Autodesk Inventor part; units mm, degrees
ref_plane "YZ Plane" through (0, 0, 0) normal (1, 0, 0) x (0, 1, 0)
ref_plane "XZ Plane" through (0, 0, 0) normal (0, 1, 0) x (-1, 0, 0)
ref_plane "XY Plane" through (0, 0, 0) normal (0, 0, 1) x (1, 0, 0)
sketch "Sketch1" plane through (0, 0, 0) normal (0, 1, 0) x (-1, 0, 0)
  line L0 (0, 0) -> (9.525, 0)
  line L1 (9.525, 0) -> (9.525, -28.575)
  line L2 (9.525, -28.575) -> (0, -28.575)
  line L3 (0, -28.575) -> (0, 0)
  circle A0 centre (3.175, -4.0894) radius 1.27
  circle A1 centre (3.175, -24.4856) radius 1.27
  dimension "d0" = 9.525
  dimension "d1" = 28.575
  dimension "d2" = 2.54
  dimension "d3" = 2.54
  dimension "d4" = 20.3962
  dimension "d5" = 4.0894
  dimension "d6" = 6.35
extrude "Extrusion1" add sketch "Sketch1" along normal blind 3.175
sketch "Sketch2" plane through (-9.525, 0, -28.575) normal (-1, 0, 0) x (0, 0, 1)
  line L0 (28.575, 0) -> (0, 0)
  line L1 (28.575, 0) -> (28.575, 3.175)
  line L2 (0, 3.175) -> (28.575, 3.175)
  line L3 (0, 0) -> (0, 3.175)
  line L4 (28.575, 3.175) -> (0, 3.175)
  line L5 (28.575, 3.175) -> (0, 3.175)
  line L6 (0, 3.175) -> (0, -6.35)
  line L7 (0, -6.35) -> (28.575, -6.35)
  line L8 (28.575, -6.35) -> (28.575, 3.175)
  point P0 (28.575, 0)
  dimension "d9" = 9.525
extrude "Extrusion2" add sketch "Sketch2" along normal blind 1.5875
sketch "Sketch3" plane through (-9.525, 0, -28.575) normal (1, 0, 0) x (0, 0, -1)
  line L0 (-28.575, 0) -> (0, 0)
  line L1 (-28.575, -6.35) -> (-28.575, 0)
  line L2 (0, -6.35) -> (-28.575, -6.35)
  line L3 (0, 0) -> (0, -6.35)
  circle A0 centre (-25.4, -3.175) radius 1.5875
  circle A1 centre (-3.175, -3.175) radius 1.5875
  point P0 (-28.575, 0)
  dimension "d12" = 3.175
  dimension "d13" = 3.175
  dimension "d14" = 3.175
  dimension "d15" = 3.175
extrude "Extrusion3" cut sketch "Sketch3" against normal blind 1.5875 contours A0 | A1
fillet "Fillet1" radius 3.175 1 edges at (-9.525, 0, -14.2875)
sketch "Sketch4" plane through (-9.525, 0, -28.575) normal (1, 0, 0) x (0, 0, -1)
  arc A0 (-4.7625, -3.175) -> (-1.5875, -3.175) centre (-3.175, -3.175) ccw
  arc A1 (-26.9875, -3.175) -> (-23.8125, -3.175) centre (-25.4, -3.175) ccw
  circle A2 centre (-25.4, -3.175) radius 3.175
  circle A3 centre (-3.175, -3.175) radius 3.175
  point P0 (-28.575, 0)
  dimension "d22" = 6.35
  dimension "d23" = 6.35
extrude "Extrusion4" cut sketch "Sketch4" along normal blind 25.4
chamfer "Chamfer2" distance 1.27 angle 45 2 edges at (-9.525, -3.175, -1.5875) (-9.525, -3.175, -23.8125)
equation "\"d3\" = d2"
equation "\"d23\" = d22"
properties part number "limitSwitchHolderMount" material "ABS Plastic"
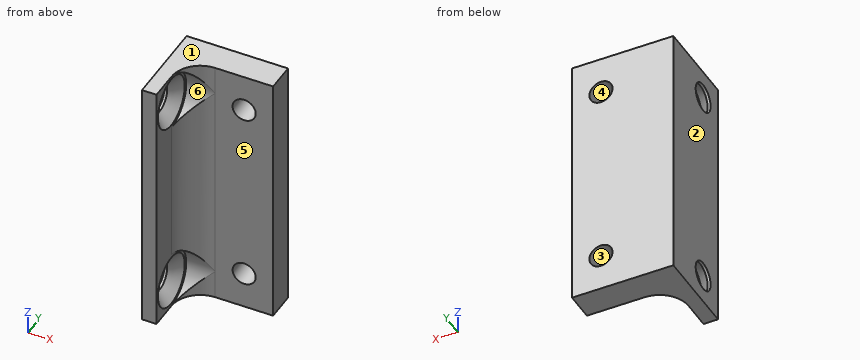
Geometry check sheet. Reference: the model listing, model coordinates, mm. Face numbers are marked on the shaded views. A direction names the side the tool comes from. Round coordinates to 2 decimals unless told otherwise and drop trailing zeros. Loops run counter-clockwise (first coordinate to the right, second up) from the corner with the lowest first, then second, coordinate; pieces in that order, holes last. Notation, with made-up numbers: (53, 55.25) - (97, 55.25) arc R8 cw to (97, 61.25) - close; hole circle Ø10 at (39.25, 76.25). An arc over 180 degrees is marked (long way). Answer as CSV lines item,"result".
(1) Cross-section at C-C, the plane y = 0.5. Enter the section's corners in (x, z) (1 decimal).
Output values:
outline,"(-11.1, -28.6) - (0, -28.6) - (0, 0) - (-11.1, 0) - close; hole circle Ø2.5 at (-3.2, -24.5); hole circle Ø2.5 at (-3.2, -4.1)"
(2) Depth check by flat-ended pin: pin 1 Ø1.5 at (x, z) = (-7.5, -24) entering from -Y; pin 2 Ø3 at (x, z) = (-3.18, -4.09) entering from +Y (3 decimals); pin 3 Ø3 at (x, z) = (-4, -7.5) entering from -Y; pin 4 Ø5 at (y, z) = (-4.5, -18) entering from +X. Enter the tip coordinate at first touch or a pass-through.
Output values:
pin 1,"stops at y = -0.55"
pin 2,"stops at y = 3.175"
pin 3,"stops at y = 0"
pin 4,"stops at x = -9.3"
(3) Set-up check for the marked faces 4, 5 and 6: record each of +Z, -Z, +X, -X, +Y, -Y from which the full face is reachable in a straight line by a thin tool's end or side.
Output values:
face 4,"+Y, -Y"
face 5,"+Z, -Z, +X, -Y"
face 6,"+X, -Y"
(4) Cross-section at B-B, the plane x = -2.5. Enter the section's corners in (y, z) (3 decimals).
Output values:
outline,"(0, -28.575) - (3.175, -28.575) - (3.175, -25.561) - (0, -25.561) - close; (0, -23.41) - (3.175, -23.41) - (3.175, -5.165) - (0, -5.165) - close; (0, -3.014) - (3.175, -3.014) - (3.175, 0) - (0, 0) - close"
(5) Cross-section at D-D, the plane x = -8. Enter the section's corners in (y, z) (3 decimals), and give its area (3 significant figures).
Output values:
outline,"(-0.462, -28.575) - (3.175, -28.575) - (3.175, 0) - (-0.462, 0) - (-0.462, -1.525) arc R3.175 cw to (-0.462, -4.825) - (-0.462, -23.75) arc R3.175 cw to (-0.462, -27.05) - close"
area,"102 mm²"
(6) Material ranges on line 1 along Z through (x, y) = (-9.75, -1.5) (3 decimals); line 2 along Z through (x, y) = (-3.5, 1.5) (3 decimals); line 3 along Y through (x, z) = (-5.75, -12.25) (3 decimals), recorded low to high.
Output values:
line 1,"z = -28.575 to -27.431, -23.369 to -5.206, -1.144 to 0"
line 2,"z = -28.575 to -25.713, -23.258 to -5.317, -2.862 to 0"
line 3,"y = 0 to 3.175"
(7) Release check for a two-part mould opening along X. For the marked faces 1, 2 and 3 record: released by +X, released by -X, zero draft, split by the parting line, or undercut.
Output values:
face 1,"zero draft"
face 2,"released by -X"
face 3,"undercut"
